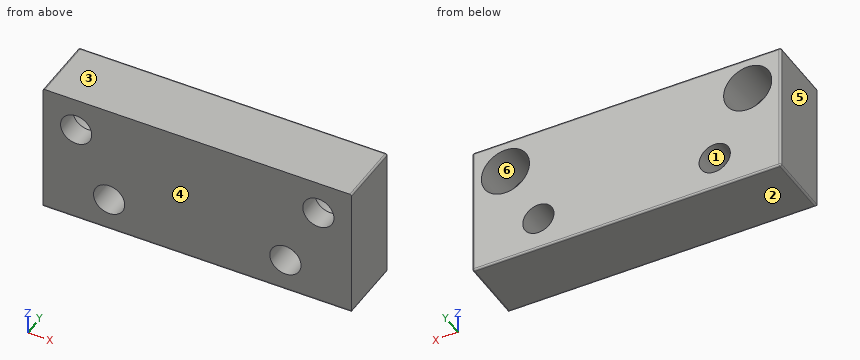
```python
from build123d import *

# Parameters (mm, degrees)
F0_W     = 44.45
F0_H     = 19.05
F0_R     = 2.2479
F0_R_2   = 3.4671
F1_DEPTH = 9.525
F2_DEPTH = 6.35
F3_R     = 0.254


with BuildPart() as f1:
    # F0 (on Front) → F1 (new body)
    with BuildSketch(Plane.XZ):
        Rectangle(F0_W, F0_H)
        with Locations((-12.7, -4.7498)):
            Circle(F0_R, mode=Mode.SUBTRACT)
        with Locations((12.7, -4.7498)):
            Circle(F0_R, mode=Mode.SUBTRACT)
        with Locations((-17.4498, 4.7625)):
            Circle(F0_R_2, mode=Mode.SUBTRACT)
        with Locations((17.4498, 4.7625)):
            Circle(F0_R_2, mode=Mode.SUBTRACT)
        with Locations((17.4498, 4.7625)):
            Circle(F0_R_2)
        with Locations((17.4498, 4.7625)):
            Circle(F0_R, mode=Mode.SUBTRACT)
        with Locations((-17.4498, 4.7625)):
            Circle(F0_R_2)
        with Locations((-17.4498, 4.7625)):
            Circle(F0_R, mode=Mode.SUBTRACT)
    extrude(amount=F1_DEPTH)

    # F0 (on Front) → F2 (cut)
    with BuildSketch(Plane.XZ):
        with Locations((17.4498, 4.7625)):
            Circle(F0_R_2)
        with Locations((17.4498, 4.7625)):
            Circle(F0_R, mode=Mode.SUBTRACT)
        with Locations((-17.4498, 4.7625)):
            Circle(F0_R_2)
        with Locations((-17.4498, 4.7625)):
            Circle(F0_R, mode=Mode.SUBTRACT)
    extrude(amount=F2_DEPTH, mode=Mode.SUBTRACT)

    # F3
    f3_edges = [f1.edges().sort_by_distance(p)[0] for p in [
        (-22.225, -4.7625, 9.525),
        (-22.225, -4.7625, -9.525),
        (22.225, -4.7625, -9.525),
        (22.225, -4.7625, 9.525),
        (0, 0, 9.525),
        (-22.225, 0, 0),
        (0, 0, -9.525),
        (22.225, 0, 0),
        (0, -9.525, -9.525),
    ]]
    fillet(f3_edges, radius=F3_R)


solid = f1.part
```
Read the model definition and answer for the solid it produces. Units are mm, in the model's axes. Face numbers are marked on the shaded views. A direction names the side the tool comes from. Give positions to 0.01 mm unless a question says otherwise; leave off trailing zeros. Order: outer loops, then holes, each group sorted by start corner. A loop starts at its lowest first (then second) coordinate and runs counter-clockwise, first axis right, second up. Notation, with made-up numbers: (63, 40.25) -> (97, 40.25) arc R10 ccw to (97, 45.25) -> close; hole circle Ø6 at (47.25, -1). An arc over 180 degrees is marked (long way). Write item = value, one per line.
1. The mould has two halves that part along Z. Classify the marked faces 1, 2, 3 and 4: +Z half, -Z half, draft (parallel to the pull), parting line (faces both ways), or undercut.
Numbers:
face_1 = undercut
face_2 = -Z half
face_3 = +Z half
face_4 = draft
2. A cutting plane is placed at D-D, the plane z = 6.5. Write down the section's boundary in (x, y) (3 decimals), and give its area (3 significant figures).
Numbers:
outline = (-22.225, -9.525) -> (-18.876, -9.525) -> (-18.876, -6.35) -> (-20.45, -6.35) -> (-20.45, 0) -> (-21.971, 0) arc R0.254 ccw to (-22.225, -0.254) -> close; (-16.024, -9.525) -> (16.024, -9.525) -> (16.024, -6.35) -> (14.449, -6.35) -> (14.449, 0) -> (-14.449, 0) -> (-14.449, -6.35) -> (-16.024, -6.35) -> close; (18.876, -9.525) -> (22.225, -9.525) -> (22.225, -0.254) arc R0.254 ccw to (21.971, 0) -> (20.45, 0) -> (20.45, -6.35) -> (18.876, -6.35) -> close
area = 329 mm²
3. Given pin 1 (6 mm diameter, centred on x = -17.45, z = 4.76, fed in from +Y), flat-ended and moving along its own axis, determine where the tip first touches the part or whether it passes through.
Numbers:
pin_1 = -6.35
4. Straight lines are drawn through the part: line 1 along X through (y, z) = (-5.5, 5) (3 decimals); line 2 along Z through (x, y) = (-12.7, -3.25) (3 decimals); line 3 along X through (y, z) = (-4.5, -6) (3 decimals). For each, find the intervals that lie inside material, in ascending order.
Numbers:
line_1 = -22.225 to -20.909, -13.991 to 13.991, 20.909 to 22.225
line_2 = -9.525 to -6.998, -2.502 to 9.525
line_3 = -22.225 to -14.568, -10.832 to 10.832, 14.568 to 22.225
5. For the marked faces 5 and 6, determine the directions among +Z, -Z, +X, -X, +Y, -Y from which every point of the face is accessible in a straight line to the end or side of a thin tool.
Numbers:
face_5 = +Z, -Z, -X, +Y, -Y
face_6 = +Y
6. A cutting plane is placed at B-B, the plane z = 3. Count the separate pieces of the cut face and the enclosed holes in it, and give its area (3 significant figures).
Numbers:
separate_pieces = 3
enclosed_holes = 0
area = 330 mm²
7. A cutting plane is placed at A-A, the plane x = -12.7. Write down the section's boundary in (y, z) (3 decimals).
Numbers:
outline = (-9.525, -9.271) arc R0.254 ccw to (-9.271, -9.525) -> (-0.254, -9.525) arc R0.254 ccw to (0, -9.271) -> (0, -6.998) -> (-9.525, -6.998) -> close; (-9.525, -2.502) -> (0, -2.502) -> (0, 9.271) arc R0.254 ccw to (-0.254, 9.525) -> (-9.525, 9.525) -> close
8. A cutting plane is placed at C-C, the plane x = 16.5. Write down the section's boundary in (y, z) (3 decimals).
Numbers:
outline = (-9.525, -9.271) arc R0.254 ccw to (-9.271, -9.525) -> (-0.254, -9.525) arc R0.254 ccw to (0, -9.271) -> (0, 1.428) -> (-6.35, 1.428) -> (-6.35, 2.725) -> (-9.525, 2.725) -> close; (-9.525, 6.8) -> (-6.35, 6.8) -> (-6.35, 8.097) -> (0, 8.097) -> (0, 9.271) arc R0.254 ccw to (-0.254, 9.525) -> (-9.525, 9.525) -> close
